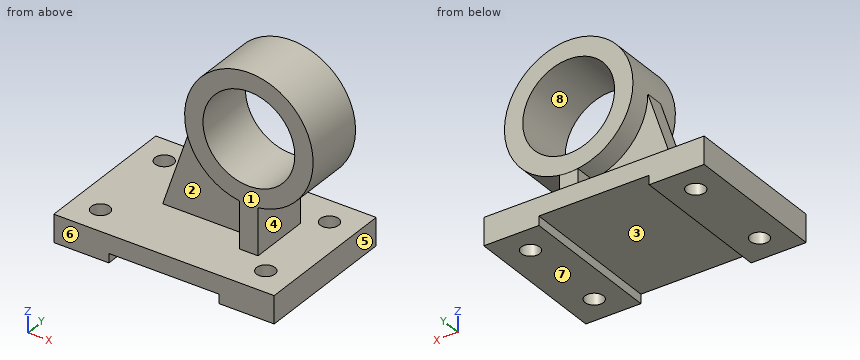
from build123d import *

# Parameters (mm, degrees)
F0_W      = 120
F0_H      = 80
F1_DEPTH  = 15
F2_W      = 60
F2_H      = 10
F3_DEPTH  = 80.001
F5_D      = 10
F7_DEPTH  = 60
F8_R      = 35
F9_DEPTH  = 33.282083
F10_R     = 25
F11_DEPTH = 56.642041
F13_DEPTH = 25


with BuildPart() as f1:
    # F0 (on Top) → F1 (new body)
    with BuildSketch(Plane.XY):
        Rectangle(F0_W, F0_H)
    extrude(amount=F1_DEPTH)

    # F2 (on face) → F3 (cut, through all)
    with BuildSketch(Plane.XZ.offset(40)):
        Rectangle(F2_W, F2_H)
    extrude(amount=-F3_DEPTH, mode=Mode.SUBTRACT)

    # F5 (through all)
    with Locations(Plane.XY.offset(15)):
        with Locations((-45, 25), (45, 25), (-45, -25), (45, -25)):
            Hole(F5_D / 2)

    # F6 (on face) → F7 (join)
    with BuildSketch(Plane.XY.offset(15)):
        Polygon((-25, -5), (25, -5), (25, -16.641041), (35, -16.641041), (35, -5), (35, 5), (35, 16.641041), (25, 16.641041), (25, 5), (-25, 5), align=None)
    extrude(amount=F7_DEPTH)

    # F8 (on face) → F9 (join, through all)
    with BuildSketch(Plane.XZ.offset(16.641041)):
        with Locations((30, 75)):
            Circle(F8_R)
    extrude(amount=-F9_DEPTH)

    # F10 (on face) → F11 (cut, through all)
    with BuildSketch(Plane.XZ.offset(16.641041)):
        with Locations((30, 75)):
            Circle(F10_R)
    extrude(amount=-F11_DEPTH, mode=Mode.SUBTRACT)

    # F12 (on face) → F13 (cut)
    with BuildSketch(Plane.XZ.offset(5)):
        Polygon((-25, 16.937228), (-25, 15), (-5, 75), (-25, 75), align=None)
    extrude(amount=-F13_DEPTH, mode=Mode.SUBTRACT)


solid = f1.part
Design review of the part built by this model. Coordinates are the model's own, in mm. Face numbers are marked on the shaded views. A direction names the side the tool comes from. Round coordinates to 2 decimals unless told otherwise and drop trailing zeros. Write each loop counter-clockwise with the first axis right and the second up, starting at its lowest first coordinate (ties: lowest second). Pieces come first, ordered by that corner, then holes. Notation, with made-up numbers: (-5.75, 40.5) -> (16.25, 40.5) arc R15 cw to (16.25, 47.5) -> close; hole circle Ø8 at (-26, 73.25). An arc over 180 degrees is marked (long way). One line per item, written item: value. Start each with the question number.
Q1. Insertion check: P1, Ø12, axis at x = 35.5, y = -4, coming from the +Z side; P2, Ø4.5, axis at y = -15, z = 4.5, coming from the +X side; P3, Ø13, axis at x = 45, y = -25, coming from the +Z side. Each pin has a flat end and moves straight along its axis. Give the tip position at first contact, or say it passes through.
Q2. To check wall thickness, follow probe 1 along Y at (x, z) = (45, 6); probe 2 along Z at (x, y) = (39.5, -15); probe 3 along Z at (x, y) = (43, -12). State the ranges of each line that lie inside material, in increasing order.
Q3. Add section D-D (y = 32.5). Give the boundary of the cut face in (x, z).
Q4. Add section C-C (z = 90). Give the boundary of the cut face in (x, y).
Q5. Add section B-B (x = -45). Give the boundary of the cut face in (y, z).
Q6. Tool access review of the marked faces 1, 2, 3, 4 and 5: name each direction out of +Z, -Z, +X, -X, +Y, -Y from which nothing blocks a thin tool from reaching the whole face with its end or side.
Q7. Add section A-A (y = 2). Give the boundary of the cut face in (x, z).
Q8. The part is to be moulded in two halves that separate along Z. For the marked faces 6, 7 and 8, say which applies: pulls with the +Z half, pulls with the -Z half, needs draft (parallel to the pull), parting line crosses it, or undercut.
Response:
1. P1: stops at z = 110
1. P2: stops at x = 60
1. P3: stops at z = 15
2. probe 1: y = -40 to -30, -20 to 20, 30 to 40
2. probe 2: z = 0 to 15, 41.31 to 51.88, 98.12 to 108.69
2. probe 3: z = 0 to 15, 42.5 to 53.65, 96.35 to 107.5
3. outline: (-60, 0) -> (-30, 0) -> (-30, 5) -> (30, 5) -> (30, 0) -> (60, 0) -> (60, 15) -> (-60, 15) -> close
4. outline: (-1.62, -16.64) -> (10, -16.64) -> (10, 16.64) -> (-1.62, 16.64) -> close; (50, -16.64) -> (61.62, -16.64) -> (61.62, 16.64) -> (50, 16.64) -> close
5. outline: (-40, 0) -> (-30, 0) -> (-30, 15) -> (-40, 15) -> close; (-20, 0) -> (20, 0) -> (20, 15) -> (-20, 15) -> close; (30, 0) -> (40, 0) -> (40, 15) -> (30, 15) -> close
6. face 1: +Z, +X, -X, -Y
6. face 2: -X, -Y
6. face 3: -Z, +Y, -Y
6. face 4: +X, +Y, -Y
6. face 5: -Z, +X, +Y, -Y
7. outline: (-60, 0) -> (-30, 0) -> (-30, 5) -> (30, 5) -> (30, 0) -> (60, 0) -> (60, 15) -> (35, 15) -> (35, 40.36) arc R35 ccw (long way) to (-5, 75) -> (-25, 15) -> (-60, 15) -> close; hole circle Ø50 at (30, 75)
8. face 6: needs draft
8. face 7: pulls with the -Z half
8. face 8: undercut
